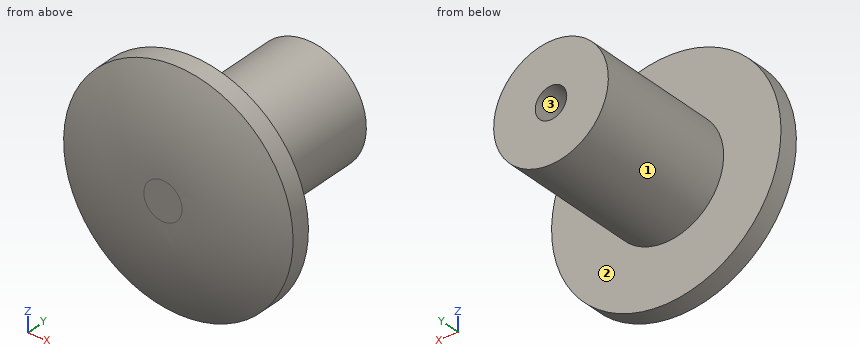
```python
from build123d import *

# Parameters (mm, degrees)
M4X0_7_TAPPED_HOLE1_D     = 3.3
M4X0_7_TAPPED_HOLE1_DEPTH = 10.1
M4X0_7_TAPPED_HOLE1_TIP   = 0.991420021


with BuildPart() as part:
    # Sketch1 → Revolve1 (revolve)
    with BuildSketch(Plane.XY, mode=Mode.PRIVATE) as revolve1_sk:
        with BuildLine():
            Line((0, 0), (-2, 0))
            ThreePointArc((-2, 0), (-7.099019514, 0.504902432), (-12, 2))
            Line((-12, 2), (-12, 4))
            Line((-12, 4), (-6, 4))
            Line((-6, 4), (-6, 19))
            Line((-6, 19), (0, 19))
            Line((0, 19), (0, 0))
        make_face()
    revolve(revolve1_sk.sketch.rotate(Axis((0, -1.785426229, 0), (0, 1, 0)), 270), axis=Axis((0, -1.785426229, 0), (0, 1, 0)))

    # M4x0.7 Tapped Hole1
    with Locations(Plane(origin=(0, 19, 0), x_dir=(1, 0, 0), z_dir=(0, 1, 0))):
        with Locations((0, 0)):
            Hole(M4X0_7_TAPPED_HOLE1_D / 2, depth=M4X0_7_TAPPED_HOLE1_DEPTH)
            with Locations((0, 0, -(M4X0_7_TAPPED_HOLE1_DEPTH + M4X0_7_TAPPED_HOLE1_TIP / 2))):  # 118° drill point
                Cone(0, M4X0_7_TAPPED_HOLE1_D / 2, M4X0_7_TAPPED_HOLE1_TIP, mode=Mode.SUBTRACT)


solid = part.part
```
The listing builds one solid part. Answer for the finished solid, in the listing's coordinates (mm). Face numbers are marked on the shaded views. Coordinates: 2 decimals unless noted, no trailing zeros. Write each loop counter-clockwise with the first axis right and the second up, starting at its lowest first coordinate (ties: lowest second). Pieces come first, ordered by that corner, then holes. Notation, with made-up numbers: (82, 43.5) - (121, 43.5) arc R14 ccw to (121, 51.5) - close; hole circle Ø7 at (53.5, 74.25). An arc over 180 degrees is marked (long way). Return JSON: item names as keys, results as strings. Group by question number.
1. Given pin 1 (10 mm diameter, centred on x = 7.5, y = 2.5, fed in from -Z); pin 2 (10 mm diameter, centred on y = 17, z = 7, fed in from -X); pin 3 (8 mm diameter, centred on x = 9, y = 11, fed in from -Z), each flat-ended and moving along its own axis, determine where each tip first touches the part or whether it passes through.
2. Determine the mould class of the marked faces 1, 2 and 3 for opening direction X: released by +X, released by -X, zero draft, split by the parting line, or undercut.
3. A cutting plane is placed at A-A, the plane y = 10.5. Determine the outline of the cut face in (x, z), plus the area to 3 significant figures.
4. Straight lines are drawn through the part: L1, parallel to Z at x = 0.25, y = 11.25; L2, parallel to X at y = 10, z = 0.75; L3, parallel to X at y = 11.25, z = -4.25. For each, find the intervals that lie inside material, in ascending order.
Ans:
{
 "1": {"pin 1": "z = -11.74", "pin 2": "x = -5.66", "pin 3": "z = -3.32"},
 "2": {"face 1": "split by the parting line", "face 2": "zero draft", "face 3": "undercut"},
 "3": {"outline": "circle Ø12 at (0, 0); hole circle Ø3.3 at (0, 0)", "area": "105 mm²"},
 "4": {"L1": "-5.99 to -1.63, 1.63 to 5.99", "L2": "-5.95 to -1.47, 1.47 to 5.95", "L3": "-4.24 to 4.24"}
}
